Input: part model. Units: mm. Frame: model coordinates. Face numbers are marked on the shaded views. A direction names the side the tool comes from. Coordinates: 2 decimals unless noted, no trailing zeros. Write each loop counter-clockwise with the first axis right and the second up, starting at its lowest first coordinate (ties: lowest second). Pieces come first, ordered by that corner, then holes.
1) Section query B-B (z = -30). Output: boundary loops of the cut face in (x, y), then the cut area to 3 significant figures.
2) Draft query along Z for the marked faces 3, 4 and 5. Return one class per face: pulls with the +Z half, pulls with the -Z half, needs draft (parallel to the pull), parting line crosses it, or undercut.
3) Pin query (flat end, axial travel): pin 1 Ø4.5 at (x, y) = (7.2, -1.66) entering from -Z; pin 2 Ø8 at (y, z) = (4.5, -17) entering from +X; pin 3 Ø8 at (x, z) = (-3.5, -10) entering from -Y; pin 4 Ø3 at (x, y) = (-4.8, -1.66) entering from +Z. Return the tip coordinate at first contact, or that it passes through.
4) Set-up query: the marked faces 1 and 2. Return all of +Z, -Z, +X, -X, +Y, -Y with unobstructed straight access to the full face (end or side cutting, diameter ignored); none if empty.
5) Line query: L1, parallel to X at y = 9, z = 2; L2, parallel to Z at x = 2.25, y = 22.5; L3, parallel to Z at x = 2.25, y = -3. Output: solid intervals per line, ascending.
6) Section query D-D (x = -5). Output: boundary loops of the cut face in (y, z).
7) Section query C-C (x = 3). Output: boundary loops of the cut face in (y, z).
8) Section query A-A (y = -1). Output: boundary loops of the cut face in (x, z).
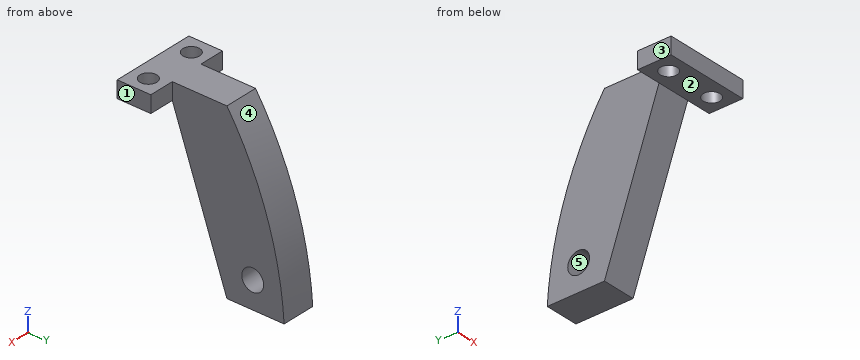
Autodesk Inventor part; units mm, degrees
ref_plane "YZ Plane" through (0, 0, 0) normal (1, 0, 0) x (0, 1, 0)
ref_plane "XZ Plane" through (0, 0, 0) normal (0, 1, 0) x (-1, 0, 0)
ref_plane "XY Plane" through (0, 0, 0) normal (0, 0, 1) x (1, 0, 0)
sketch "Sketch1" plane through (0, 0, 0) normal (0, 0, 1) x (1, 0, 0)
  line L0 (-8.802, 2.3397) -> (11.198, 2.3397)
  line L1 (11.198, 2.3397) -> (11.198, -5.6603)
  line L2 (11.198, -5.6603) -> (-8.802, -5.6603)
  line L3 (-8.802, -5.6603) -> (-8.802, 2.3397)
  circle A0 centre (-4.802, -1.6603) radius 2
  circle A1 centre (7.198, -1.6603) radius 2
  point P0 (0, 0)
  dimension "d4" = 4
  dimension "d0" = 4
  dimension "d1" = 4
  dimension "d2" = 12
  dimension "d3" = 4
  dimension "d5" = 4
  dimension "d7" = 8
  dimension "d8" = 4
  dimension "d9" = 20
  dimension "d10" = 4
extrude "Extrusion1" add sketch "Sketch1" along normal blind 4
ref_plane "Work Plane1" through (1.198, -5.6603, 0) normal (1, 0, 0) x (0, 0, -1)
sketch "Sketch2" plane through (1.198, -5.6603, 0) normal (1, 0, 0) x (0, 0, -1)
  arc A0 (36.9246, 34.6197) -> (-4, 21) centre (41.9479, -48.7697) ccw
  line L0 (0, 0) -> (0, 8)
  line L1 (36.9247, 21) -> (36.9246, 34.6197)
  arc A1 (44.549, 70.6711) -> (-44.2597, 70.8526) centre (0, 0) ccw
  circle A2 centre (9.9821, 76.8133) radius 2.6
  line L2 (9.9821, 96.2846) -> (9.9821, 47.2392) construction
  line L3 (62.1306, 76.8133) -> (-24.9977, 76.8133) construction
  line L4 (0, 0) -> (0, 8) construction
  circle A3 centre (30.5669, 27.142) radius 2.6
  line L5 (-4, 0) -> (-4, 8)
  line L6 (0, 8) -> (-4, 8)
  line L7 (36.9247, 21) -> (0, 8)
  line L8 (0, 8) -> (-4, 8)
  line L9 (36.9247, 21) -> (-4, 21) construction
  line L10 (-4, 21) -> (-4, 8)
  point P0 (0, 5.6603)
  dimension "d15" = 34.5669
  dimension "d16" = 6.1422
  dimension "d17" = 34.5669
  dimension "d22" = 13.6197
  dimension "d27" = 5.2
  dimension "d32" = 6.142
  dimension "d33" = 13
extrude "Extrusion4" add sketch "Sketch2" along normal mid plane 8 contours L1 L7 L6 L10 A0
sketch "Sketch3" plane through (0, 0, 4) normal (0, 0, 1) x (1, 0, 0)
  circle A0 centre (7.198, -1.6603) radius 2
  circle A1 centre (-4.802, -1.6603) radius 2
  line L0 (-8.802, 2.3397) -> (-8.802, -5.6603)
  line L1 (-8.802, -5.6603) -> (11.198, -5.6603)
  circle A2 centre (1.198, -1.6603) radius 0.6445
  point P0 (0, 0)
  dimension "d28" = 12
  dimension "d29" = 6
  dimension "d30" = 8
  dimension "d31" = 4
equation "\"d4\" = d3"
equation "\"d3\" = d8"
equation "\"d5\" = d4"
properties part number "motor_elytra_interface" material "Nylon 6/6"
Answer:
1. outline: (-2.8, 12.9) - (5.2, 12.9) - (5.2, 18.94) - (-2.8, 18.94) - close; (-2.8, 24.02) - (5.2, 24.02) - (5.2, 28.25) - (-2.8, 28.25) - close
1. area: 82.2 mm2
2. face 3: needs draft
2. face 4: pulls with the +Z half
2. face 5: undercut
3. pin 1: stops at z = 0
3. pin 2: stops at x = 5.2
3. pin 3: stops at y = 4.47
3. pin 4: passes through
4. face 1: +Z, -Z, +X, +Y, -Y
4. face 2: -Z, +X, -X, -Y
5. L1: x = -2.8 to 5.2
5. L2: z = -36.92 to -32.96, -28.17 to -9.38
5. L3: z = 0 to 4
6. outline: (-5.66, 0) - (-3.65, 0) - (-3.65, 4) - (-5.66, 4) - close; (0.33, 0) - (2.34, 0) - (2.34, 4) - (0.33, 4) - close
7. outline: (-5.66, 0) - (2.34, 0) - (15.34, -36.92) - (28.96, -36.92) arc R83.54 ccw to (15.34, 4) - (-5.66, 4) - close; hole circle Ø5.2 at (21.48, -30.57)
8. outline: (-8.8, 0) - (-6.69, 0) - (-6.69, 4) - (-8.8, 4) - close; (-2.91, 0) - (5.31, 0) - (5.31, 4) - (-2.91, 4) - close; (9.09, 0) - (11.2, 0) - (11.2, 4) - (9.09, 4) - close
